Read the model definition and answer for the solid it produces. Units are mm, in the model's axes. Round coordinates to 2 decimals unless told otherwise and drop trailing zeros. Write each loop counter-clockwise with the first axis right and the second up, starting at its lowest first coordinate (ties: lowest second). Pieces come first, ordered by that corner, then holes. Notation, with made-up numbers: (73, -8) -> (124, -8) arc R32 cw to (124, 30) -> close; hole circle Ø5 at (77, 6). An arc over 180 degrees is marked (long way). Return JSON: item names as keys, results as strings.
from build123d import *

# Parameters (mm, degrees)
FILLET1_R          = 3.175
SKETCH2_R          = 3.175
CUT_EXTRUDE1_DEPTH = 61.491874454
CIRPATTERN1_COUNT  = 6
SCALE1_SCALE       = 0.5


with BuildPart() as part:
    # Sketch1 → Revolve1 (revolve)
    with BuildSketch(Plane(origin=(0, 0, 0), x_dir=(0, 0, -1), z_dir=(1, 0, 0)), mode=Mode.PRIVATE) as revolve1_sk:
        Polygon((0, 7.9375), (0, 41.275), (-3.175, 41.275), (-3.175, 12.7), (-19.05, 12.7), (-19.05, 7.9375), align=None)
    revolve(revolve1_sk.sketch.rotate(Axis((0, 0, 0), (0, 0, 1)), 90), axis=Axis((0, 0, 0), (0, 0, 1)))

    # Fillet1
    fillet1_edges = [part.edges().sort_by_distance(p)[0] for p in [
        (12.7, 0, 3.175),
    ]]
    fillet(fillet1_edges, radius=FILLET1_R)

    # Sketch2 → Cut-Extrude1 (cut, through all)
    with BuildSketch(Plane.XY.offset(3.175)):
        with Locations((34.925, 0)):
            Circle(SKETCH2_R)
    cut_extrude1 = extrude(amount=-CUT_EXTRUDE1_DEPTH, mode=Mode.SUBTRACT)

    # CirPattern1: Cut-Extrude1 ×6 about axis
    cirpattern1_axis = Axis((0, 0, 0), (0, 0, 1))
    for i in range(1, CIRPATTERN1_COUNT):
        add(cut_extrude1.rotate(cirpattern1_axis, i * 360 / CIRPATTERN1_COUNT), mode=Mode.SUBTRACT)


with BuildPart() as part_1:
    # Scale1: scaled about (0, 0, 3.84726884)
    add(part.part.scale(SCALE1_SCALE).moved(Location((0, 0, 1.92363442))))


solid = part_1.part
Item 1: Section B-B (y = -16) is taken. Give the vertices of the cut face in (x, z), then the cut area to 3 significant figures.
Worked answers:
{"outline": "(-13.03, 1.92) -> (-10.05, 1.92) -> (-10.05, 3.51) -> (-13.03, 3.51) -> close; (-7.41, 1.92) -> (7.41, 1.92) -> (7.41, 3.51) -> (-7.41, 3.51) -> close; (10.05, 1.92) -> (13.03, 1.92) -> (13.03, 3.51) -> (10.05, 3.51) -> close", "area": "33.0 mm2"}
Item 2: Flat-ended cylindrical pins translate along their axes: pin 1 (3 mm diameter, centred on y = 5, z = 10, fed in from +X); pin 2 (3.5 mm diameter, centred on x = -8.73, y = -15.12, fed in from +Z); pin 3 (12.5 mm diameter, centred on x = 0, y = 0, fed in from -Z). Find the tip coordinate at first contact, or state that the pin passes through.
Worked answers:
{"pin 1": "stops at x = 5.3", "pin 2": "stops at z = 3.51", "pin 3": "stops at z = 1.92"}
Item 3: Section D-D (x = -17) is taken. Give the vertices of the cut face in (y, z), then the cut area to 3 significant figures.
Worked answers:
{"outline": "(-11.7, 1.92) -> (-1.52, 1.92) -> (-1.52, 3.51) -> (-11.7, 3.51) -> close; (1.52, 1.92) -> (11.7, 1.92) -> (11.7, 3.51) -> (1.52, 3.51) -> close", "area": "32.3 mm2"}
Item 4: For a pull along Y with two mould halves and no side action, classify faces 1 (the cylindrical face through (18.977, 0.477, 2.728)), 2 (the flat face through (0, 9, 3.511)), 3 (the cylindrical face through (5.04, 3.86, 8.32)) as released by +Y, released by -Y, zero draft, split by the parting line, or undercut.
Worked answers:
{"face 1": "undercut", "face 2": "zero draft", "face 3": "split by the parting line"}
Item 5: Section C-C (y = 0) is taken. State how many separate pieces and enclosed holes the cut face has, then the cut area to 3 significant figures.
Worked answers:
{"separate pieces": "4", "enclosed holes": "0", "area": "81.7 mm2"}
Item 6: Straight lines are drawn through the part: L1, parallel to Y at x = 0, z = 5.75; L2, parallel to Z at x = 4, y = -16; L3, parallel to Y at x = 2, z = 4. For each, find the intervals that lie inside material, in ascending order. Write a range as [from, to].
Worked answers:
{"L1": "y = [-6.35, -3.97], [3.97, 6.35]", "L2": "z = [1.92, 3.51]", "L3": "y = [-6.49, -3.43], [3.43, 6.49]"}
